```python
from build123d import *

# Parameters (mm, degrees)
SKETCH1_R           = 1.6
BOSS_EXTRUDE1_DEPTH = 9
FILLET1_R           = 3
SKETCH2_R           = 5.1
CUT_EXTRUDE1_DEPTH  = 10


with BuildPart() as part:
    # Sketch1 → Boss-Extrude1 (new body)
    with BuildSketch(Plane.XY):
        with BuildLine():
            Line((-46.324821937, 10), (-42.656212912, 12.5))
            ThreePointArc((-42.656212912, 12.5), (0, 44.45), (42.656212912, 12.5))
            Line((42.656212912, 12.5), (46.324821937, 10))
            ThreePointArc((46.324821937, 10), (47.45, 0), (46.324821937, -10))
            Line((46.324821937, -10), (42.656212912, -12.5))
            ThreePointArc((42.656212912, -12.5), (0, -44.45), (-42.656212912, -12.5))
            Line((-42.656212912, -12.5), (-46.324821937, -10))
            ThreePointArc((-46.324821937, -10), (-47.45, 0), (-46.324821937, 10))
        make_face()
        with Locations((0, 41.275)):
            Circle(SKETCH1_R, mode=Mode.SUBTRACT)
        with Locations((35.745198541, 20.6375)):
            Circle(SKETCH1_R, mode=Mode.SUBTRACT)
        with Locations((35.745198541, -20.6375)):
            Circle(SKETCH1_R, mode=Mode.SUBTRACT)
        with Locations((0, -41.275)):
            Circle(SKETCH1_R, mode=Mode.SUBTRACT)
        with Locations((-35.745198541, -20.6375)):
            Circle(SKETCH1_R, mode=Mode.SUBTRACT)
        with Locations((-35.745198541, 20.6375)):
            Circle(SKETCH1_R, mode=Mode.SUBTRACT)
    extrude(amount=BOSS_EXTRUDE1_DEPTH)

    # Fillet1
    fillet1_edges = [part.edges().sort_by_distance(p)[0] for p in [
        (46.324821937, -10, 4.5),
        (42.656212912, -12.5, 4.5),
        (-42.656212912, -12.5, 4.5),
        (-46.324821937, -10, 4.5),
        (-46.324821937, 10, 4.5),
        (-42.656212912, 12.5, 4.5),
        (42.656212912, 12.5, 4.5),
        (46.324821937, 10, 4.5),
    ]]
    fillet(fillet1_edges, radius=FILLET1_R)

    # Sketch2 → Cut-Extrude1 (cut, through all)
    with BuildSketch(Plane.XY.offset(9)):
        with Locations((0, 21)):
            Circle(SKETCH2_R)
        with Locations((18.186533479, 10.5)):
            Circle(SKETCH2_R)
        with Locations((18.186533479, -10.5)):
            Circle(SKETCH2_R)
        with Locations((0, -21)):
            Circle(SKETCH2_R)
        with Locations((-18.186533479, -10.5)):
            Circle(SKETCH2_R)
        with Locations((-18.186533479, 10.5)):
            Circle(SKETCH2_R)
        Circle(SKETCH2_R)
    extrude(amount=-CUT_EXTRUDE1_DEPTH, mode=Mode.SUBTRACT)


solid = part.part
```
Here's how the part is built. I have some questions about the finished solid (model axes, mm). Coordinates: 2 decimals unless noted, no trailing zeros. Order: outer loops, then holes, each group sorted by start corner. A loop starts at its lowest first (then second) coordinate and runs counter-clockwise, first axis right, second up. Notation, with made-up numbers: M -19,4 L -6,4 A26 cw -6,42 Z; hole C 70.5,-30.75 d10. An arc over 180 degrees is marked long. Answer as a JSON object with one key per item and string values. Group by question number.
(1) Suppose I cut it at A-A, the plane x = 0. Please give me the cut outline in (y, z) (3 decimals), then the cut area to 3 significant figures.
(2) I need wall thicknesses on probe 1 along Y at (x, z) = (0, 3.75) (3 decimals); probe 2 along Y at (x, z) = (-14, 6.5); probe 3 along Y at (x, z) = (-2.5, 3). Which ranges of each line are inside material? Lowest first, please.
(3) For pin 1 (2 mm diameter, centred on y = -4, z = 6, fed in from -X); pin 2 (9 mm diameter, centred on x = 18.19, y = 10.5, fed in from -Z); pin 3 (4 mm diameter, centred on y = 21, z = 5.5, fed in from -X); pin 4 (1.5 mm diameter, centred on y = -1, z = 5.5, fed in from +X), each with a flat end and sliding along its axis, tell me the tip position at first contact or that it passes through.
(4) If we mould it in two halves opening along Y, with no side actions, what happens to faces 1 (the face through (37.2, -21.3, 4.4)), 2 (the face through (1, -9, 9)), 3 (the face through (-0.786, 44.443, 4.437))? For each: released by +Y, released by -Y, zero draft, split by the parting line, or undercut.
(5) Suppose I cut it at B-B, the plane y = 0. Please give me the cut outline in (x, z), then the cut area to 3 significant figures.
(6) Suppose I cut it at C-C, the plane z = 1.75. State how many separate pieces and enclosed holes the cut face has, then the cut area to 3 significant figures.
(7) Suppose I cut it at D-D, the plane x = -22. Please give me the cut outline in (y, z), then the cut area to 3 significant figures.
Values found:
{
 "1": {"outline": "M -44.45,0 L -42.875,0 L -42.875,9 L -44.45,9 Z; M -39.675,0 L -26.1,0 L -26.1,9 L -39.675,9 Z; M -15.9,0 L -5.1,0 L -5.1,9 L -15.9,9 Z; M 5.1,0 L 15.9,0 L 15.9,9 L 5.1,9 Z; M 26.1,0 L 39.675,0 L 39.675,9 L 26.1,9 Z; M 42.875,0 L 44.45,0 L 44.45,9 L 42.875,9 Z", "area": "467 mm^2"},
 "2": {"probe 1": "y = -44.45 to -42.875, -39.675 to -26.1, -15.9 to -5.1, 5.1 to 15.9, 26.1 to 39.675, 42.875 to 44.45", "probe 2": "y = -42.19 to -13.41, -7.59 to 7.59, 13.41 to 42.19", "probe 3": "y = -44.38 to -25.45, -16.55 to -4.45, 4.45 to 16.55, 25.45 to 44.38"},
 "3": {"pin 1": "stops at x = -47.35", "pin 2": "passes through", "pin 3": "stops at x = -40.18", "pin 4": "stops at x = 47.45"},
 "4": {"face 1": "undercut", "face 2": "zero draft", "face 3": "released by +Y"},
 "5": {"outline": "M -47.45,0 L -5.1,0 L -5.1,9 L -47.45,9 Z; M 5.1,0 L 47.45,0 L 47.45,9 L 5.1,9 Z", "area": "762 mm^2"},
 "6": {"separate pieces": "1", "enclosed holes": "13", "area": "5,720 mm^2"},
 "7": {"outline": "M -38.62,0 L -13.89,0 L -13.89,9 L -38.62,9 Z; M -7.11,0 L 7.11,0 L 7.11,9 L -7.11,9 Z; M 13.89,0 L 38.62,0 L 38.62,9 L 13.89,9 Z", "area": "573 mm^2"}
}
